from build123d import *

# Parameters (mm, degrees)
SKETCH_1_R          = 7.5
EXTRUDE_1_DEPTH     = 1
SKETCH_2_R          = 3
EXTRUDE_2_DEPTH     = 4
CUT_EXTRUDE_1_REACH = 13.726
SKETCH_3_R          = 2
CHAMFER_1_SIZE      = 0.5
FILLET_1_R          = 0.2


with BuildPart() as part:
    # 草图1 → 凸台-拉伸1 (new body)
    with BuildSketch(Plane(origin=(0, 0, 0), x_dir=(1, 0, 0), z_dir=(0, 1, 0))):
        with Locations(Location((0, 0, 0), (0, 0, 270))):
            Circle(SKETCH_1_R)
    extrude(amount=EXTRUDE_1_DEPTH)

    # 草图2 → 凸台-拉伸2 (add)
    with BuildSketch(Plane(origin=(0, 1, 0), x_dir=(1, 0, 0), z_dir=(0, 1, 0))):
        with Locations(Location((0, 0, 0), (0, 0, 270))):
            Circle(SKETCH_2_R)
    extrude(amount=EXTRUDE_2_DEPTH)

    # 草图3 → 切除-拉伸1 (cut, up to next)
    with BuildSketch(Plane(origin=(0, 5, 0), x_dir=(1, 0, 0), z_dir=(0, 1, 0)), mode=Mode.PRIVATE) as cut_extrude_1_sk1:
        with Locations(Location((0, 0, 0), (0, 0, 270))):
            Circle(SKETCH_3_R)
    cut_extrude_1_tool1 = extrude(cut_extrude_1_sk1.sketch, amount=-CUT_EXTRUDE_1_REACH, mode=Mode.PRIVATE) & part.part
    add(cut_extrude_1_tool1.solids().sort_by_distance((0, 5, 0))[0], mode=Mode.SUBTRACT)

    # 倒角1
    chamfer_1_edges = [part.edges().sort_by_distance(p)[0] for p in [
        (0, 5, -2),
        (0, 0, -2),
    ]]
    chamfer(chamfer_1_edges, length=CHAMFER_1_SIZE)

    # 圆角1
    fillet_1_edges = [part.edges().sort_by_distance(p)[0] for p in [
        (0, 0, -7.5),
        (0, 1, -7.5),
    ]]
    fillet(fillet_1_edges, radius=FILLET_1_R)


solid = part.part
Verification items for the finished model (mm, model axes). Round coordinates to 2 decimals unless told otherwise and drop trailing zeros. Order: outer loops, then holes, each group sorted by start corner. A loop starts at its lowest first (then second) coordinate and runs counter-clockwise, first axis right, second up. Notation, with made-up numbers: (-40, 19.25) -> (-18, 19.25) arc R22 cw to (-18, 40.25) -> close; hole circle Ø3 at (28.5, 52). An arc over 180 degrees is marked (long way). Put each result on its own line as item: value.
1) Material ranges on line 1 (X direction, y = 3.55, z = 0); line 2 (Y direction, x = 2.5, z = -1.75); line 3 (Z direction, x = -1.5, y = 2.3), recorded low to high.
Final values:
line 1: x = -3 to -2, 2 to 3
line 2: y = 0 to 1
line 3: z = -2.6 to -1.32, 1.32 to 2.6
2) Section check A-A (z = 0). Record the cut outline in (x, y).
Final values:
outline: (-7.5, 0.2) arc R0.2 ccw to (-7.3, 0) -> (-2.5, 0) -> (-2, 0.5) -> (-2, 4.5) -> (-2.5, 5) -> (-3, 5) -> (-3, 1) -> (-7.3, 1) arc R0.2 ccw to (-7.5, 0.8) -> close; (2, 0.5) -> (2.5, 0) -> (7.3, 0) arc R0.2 ccw to (7.5, 0.2) -> (7.5, 0.8) arc R0.2 ccw to (7.3, 1) -> (3, 1) -> (3, 5) -> (2.5, 5) -> (2, 4.5) -> close
3) Depth check by flat-ended pin: pin 1 (1 mm diameter, centred on x = -1.5, y = 0.5, fed in from +Z); pin 2 (1 mm diameter, centred on x = -1.5, y = 2.5, fed in from -Z); pin 3 (3 mm diameter, centred on y = 3, z = -2, fed in from -X); pin 4 (2.5 mm diameter, centred on x = 0, z = 0, fed in from -Y). Enter the tip coordinate at first touch or a pass-through.
Final values:
pin 1: stops at z = 7.43
pin 2: stops at z = -2.83
pin 3: stops at x = -2.96
pin 4: passes through
4) Mould release check, pull along X, two halves, no side actions. Record for faces 1 (the flat face through (-3, 1, 2)), 2 (the cylindrical face through (-2, 3, 0)), 3 (the cylindrical face through (0.9, 2.97, 2.86)): +X half, -X half, draft (parallel to the pull), parting line (faces both ways), or undercut.
Final values:
face 1: draft
face 2: undercut
face 3: parting line
5) Section check C-C (y = 1.55). Record the cut outline in (x, z), then the cut area to 3 significant figures.
Final values:
outline: circle Ø6 at (0, 0); hole circle Ø4 at (0, 0)
area: 15.7 mm^2
6) Section check B-B (x = 0). Record the cut outline in (y, z), then the cut area to 3 significant figures.
Final values:
outline: (0, -7.3) arc R0.2 ccw to (0.2, -7.5) -> (0.8, -7.5) arc R0.2 ccw to (1, -7.3) -> (1, -3) -> (5, -3) -> (5, -2.5) -> (4.5, -2) -> (0.5, -2) -> (0, -2.5) -> close; (0, 2.5) -> (0.5, 2) -> (4.5, 2) -> (5, 2.5) -> (5, 3) -> (1, 3) -> (1, 7.3) arc R0.2 ccw to (0.8, 7.5) -> (0.2, 7.5) arc R0.2 ccw to (0, 7.3) -> close
area: 18.5 mm^2
